from build123d import *

# Parameters (mm, degrees)
F0_W     = 76.2
F0_H     = 38.1
F1_DEPTH = 25.4
F2_R     = 11.1125
F3_DEPTH = 12.7
F4_SIZE  = 3.175
F5_T     = 7.9375
F6_R     = 3.175
F7_DEPTH = 7.9375
F8_R     = 3.0126564395
F9_DEPTH = 7.9375


# Not quite as in the source:
# - a shell that OpenCascade refuses in one call is made with other operations: the cavity is built on its own and cut out


with BuildPart() as f1:
    # F0 (on Top) → F1 (new body)
    with BuildSketch(Plane.XY):
        with Locations((-5.8783623338, 3.9097142845)):
            Rectangle(F0_W, F0_H)
    extrude(amount=F1_DEPTH)

    # F2 (on face) → F3 (join)
    with BuildSketch(Plane.XY.offset(25.4)):
        with Locations((-24.9283623338, 3.9097142845)):
            Circle(F2_R)
        with Locations((13.1716376662, 3.9097142845)):
            Circle(F2_R)
    extrude(amount=F3_DEPTH)

    # F4
    f4_edges = [f1.edges().sort_by_distance(p)[0] for p in [
        (-36.040862, 3.909714, 38.1),
        (2.059138, 3.909714, 38.1),
        (32.221638, 3.909714, 25.4),
        (-5.878362, 22.959714, 25.4),
        (-43.978362, 3.909714, 25.4),
        (-5.878362, -15.140286, 25.4),
    ]]
    chamfer(f4_edges, length=F4_SIZE)

    # F5: shell of thickness 7.9375, made by hand


with BuildPart() as f5_core1:
    # F5_t2: copy of F1
    add(f1.part)

    # the walls: a layer under each face that stays
    f5_faces = [f5_core1.faces().sort_by_distance(p)[0] for p in [
        (32.2216376662, 3.9097142845, 11.1125),
        (-5.8783623338, -15.1402857155, 11.1125),
        (30.6341376662, 3.9097142845, 23.8125),
        (-5.8783623338, 22.9597142845, 11.1125),
        (-43.9783623338, 3.9097142845, 11.1125),
        (-5.8783623338, -13.5527857155, 23.8125),
        (-5.8783623338, 3.9097142845, 25.4),
        (-5.8783623338, 21.3722142845, 23.8125),
        (-42.3908623338, 3.9097142845, 23.8125),
        (-36.0408623338, 3.9097142845, 30.1625),
        (2.0591376662, 3.9097142845, 30.1625),
        (-34.4533623338, 3.9097142845, 36.5125),
        (3.6466376662, 3.9097142845, 36.5125),
        (-24.9283623338, 3.9097142845, 38.1),
        (13.1716376662, 3.9097142845, 38.1),
    ]]
    thicken(f5_faces, amount=-F5_T, mode=Mode.SUBTRACT)

    # F5_s3 → F5_t4 (revolve, cut)
    with BuildSketch(Plane.XZ.offset(-3.9097142845)):
        Polygon((-13.7364873338, 25.479375), (-13.8158623338, 17.4625), (-21.7533623338, 17.4625), (-21.7533623338, 25.4), align=None)
    revolve(axis=Axis((-24.9283623338, 3.9097142845, 25.4), (0, 0, 1)), mode=Mode.SUBTRACT)

    # F5_s5 → F5_t6 (revolve, cut)
    with BuildSketch(Plane.XZ.offset(-3.9097142845)):
        Polygon((24.3635126662, 25.479375), (24.2841376662, 17.4625), (16.3466376662, 17.4625), (16.3466376662, 25.4), align=None)
    revolve(axis=Axis((13.1716376662, 3.9097142845, 25.4), (0, 0, 1)), mode=Mode.SUBTRACT)


with BuildPart() as f1_1:
    add(f1.part)

    # what is left inside the walls is the cavity
    f5_cavity = [f5_core1.part.solids().sort_by_distance(p)[0] for p in [
        (-5.878362, 0.205548, 0.079375),
    ]]
    add(f5_cavity, mode=Mode.SUBTRACT)

    # F6 (on face) → F7 (cut)
    with BuildSketch(Plane.XZ.offset(15.1402857155)):
        with Locations((-5.8783623338, 12.7)):
            Circle(F6_R)
    extrude(amount=-F7_DEPTH, mode=Mode.SUBTRACT)

    # F8 (on face) → F9 (cut)
    with BuildSketch(Plane(origin=(0, 22.9597142845, 0), x_dir=(-1, 0, 0), z_dir=(0, 1, 0))):
        with Locations((5.8783623338, 12.7)):
            Circle(F8_R)
    extrude(amount=-F9_DEPTH, mode=Mode.SUBTRACT)


solid = f1_1.part
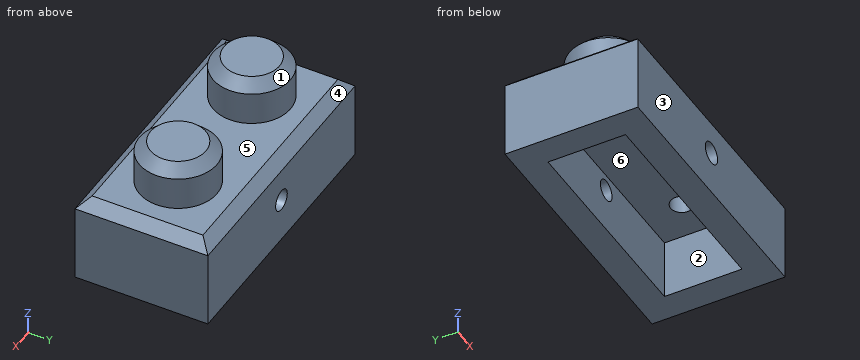
Model file for the job. Use its own axes, mm. Face numbers are marked on the shaded views. A direction names the side the tool comes from. Coordinates: 2 decimals unless noted, no trailing zeros. Order: outer loops, then holes, each group sorted by start corner. A loop starts at its lowest first (then second) coordinate and runs counter-clockwise, first axis right, second up. Notation, with made-up numbers: M -24,79.5 L -16,79.5 A29 cw -16,103.5 Z; hole C 36.25,58 d5. An arc over 180 degrees is marked long. Return JSON: item names as keys, results as strings.
1. Pull direction Y, two halves, no side cores. Call the marked faces 1, 2 and 3: +Y half, -Y half, draft (parallel to the pull), parting line (faces both ways), or undercut.
Ans:
{"face 1": "parting line", "face 2": "undercut", "face 3": "-Y half"}
2. Tool access for the marked faces 4, 5 and 6: list every direction of +Z, -Z, +X, -X, +Y, -Y with a clear straight run to the whole face (end or side of a thin tool).
Ans:
{"face 4": "+Z, +X, -X, +Y", "face 5": "+Z", "face 6": "-Z"}
3. Saw through at C-C (x = -0.5). Give the cut face in (y, z) (1 decimal).
Ans:
{"outline": "M -15.1,0 L -7.2,0 L -7.2,17.5 L 15,17.5 L 15,0 L 23,0 L 23,22.2 L 19.8,25.4 L -12,25.4 L -15.1,22.2 Z"}
4. Saw through at A-A (y = -8). Give the cut face in (x, z) (3 decimals).
Ans:
{"outline": "M -43.978,0 L 32.222,0 L 32.222,22.225 L 29.047,25.4 L -40.803,25.4 L -43.978,22.225 Z; hole C -5.878,12.7 d6.35"}
5. Flat gauge pins, fed straight in: pin 1 (4 mm diameter, centred on x = -15.5, y = 8.5, fed in from +Z); pin 2 (5 mm diameter, centred on x = -23.5, y = 3.5, fed in from -Z); pin 3 (1.5 mm diameter, centred on x = -30.5, z = 32.5, fed in from +Y). Where does each tip first touch, or does it go through?
Ans:
{"pin 1": "z = 37.55", "pin 2": "z = 17.46", "pin 3": "y = 13.92"}
6. Saw through at D-D (z = 26.5). Give the number of separate pieces and of enclosed holes in the cut face, and give its area (3 significant figures).
Ans:
{"separate pieces": "2", "enclosed holes": "2", "area": "713 mm^2"}
7. Drill centre lines: probe 1 along X at (y, z) = (13, 15.5); probe 2 along Y at (x, z) = (-13.5, 16.5); probe 3 along Z at (x, y) = (18, 18). Where is each one in solid material? Low to high.
Ans:
{"probe 1": "-43.98 to -36.04, 24.28 to 32.22", "probe 2": "-15.14 to -7.2, 15.02 to 22.96", "probe 3": "0 to 25.4"}
8. Saw through at B-B (z = 12.7). Give the cut face in (x, y).
Ans:
{"outline": "M -43.98,-15.14 L -9.05,-15.14 L -9.05,-7.2 L -36.04,-7.2 L -36.04,15.02 L -8.89,15.02 L -8.89,22.96 L -43.98,22.96 Z; M -2.87,15.02 L 24.28,15.02 L 24.28,-7.2 L -2.7,-7.2 L -2.7,-15.14 L 32.22,-15.14 L 32.22,22.96 L -2.87,22.96 Z"}
